Read the model definition and answer for the solid it produces. Units are mm, in the model's axes. Face numbers are marked on the shaded views. Coordinates: 2 decimals unless noted, no trailing zeros. Write each loop counter-clockwise with the first axis right and the second up, starting at its lowest first coordinate (ties: lowest second). Pieces come first, ordered by that corner, then holes. Notation, with made-up numbers: (0, 2) - (7, 2) arc R10 ccw to (7, 15) - close; hole circle Ø4 at (-37.5, 27). An arc over 180 degrees is marked (long way). Return JSON: item names as keys, results as strings.
```python
from build123d import *

# Parameters (mm, degrees)
SKETCH_1_R      = 5.5
EXTRUDE_1_DEPTH = 1.5
SKETCH_2_R      = 2.5
EXTRUDE_2_DEPTH = 2
SKETCH_3_R      = 10.188778254
EXTRUDE_3_DEPTH = 20
FILLET_2_R      = 2
FILLET_3_R      = 2
SCALE_1_SCALE   = 1.703703703


with BuildPart() as part:
    # 草图1 → 凸台-拉伸1 (new body)
    with BuildSketch(Plane(origin=(0, 0, 0), x_dir=(1, 0, 0), z_dir=(0, 1, 0))):
        with Locations(Location((0, 0, 0), (0, 0, 270))):
            Circle(SKETCH_1_R)
    extrude(amount=EXTRUDE_1_DEPTH)

    # 草图2 → 凸台-拉伸2 (add)
    with BuildSketch(Plane(origin=(0, 1.5, 0), x_dir=(1, 0, 0), z_dir=(0, 1, 0))):
        with Locations(Location((0, 0, 0), (0, 0, 270))):
            Circle(SKETCH_2_R)
    extrude(amount=EXTRUDE_2_DEPTH)

    # 草图3 → 凸台-拉伸3 (add)
    with BuildSketch(Plane(origin=(0, 3.5, 0), x_dir=(1, 0, 0), z_dir=(0, 1, 0))):
        with Locations(Location((0, 0, 0), (0, 0, 270))):
            Circle(SKETCH_3_R)
    extrude(amount=EXTRUDE_3_DEPTH)

    # 圆角2
    fillet_2_edges = [part.edges().sort_by_distance(p)[0] for p in [
        (0, 23.5, -10.188778254),
    ]]
    fillet(fillet_2_edges, radius=FILLET_2_R)

    # 圆角3
    fillet_3_edges = [part.edges().sort_by_distance(p)[0] for p in [
        (0, 3.5, -2.5),
        (0, 3.5, -10.188778254),
    ]]
    fillet(fillet_3_edges, radius=FILLET_3_R - 0.0001)  # a hair under: the kernel refuses the full size


with BuildPart() as part_1:
    # 缩放比例1: scaled about (0, 13.134921616, 0)
    add(part.part.scale(SCALE_1_SCALE).moved(Location((0, -9.243092979, 0))))


solid = part_1.part
```
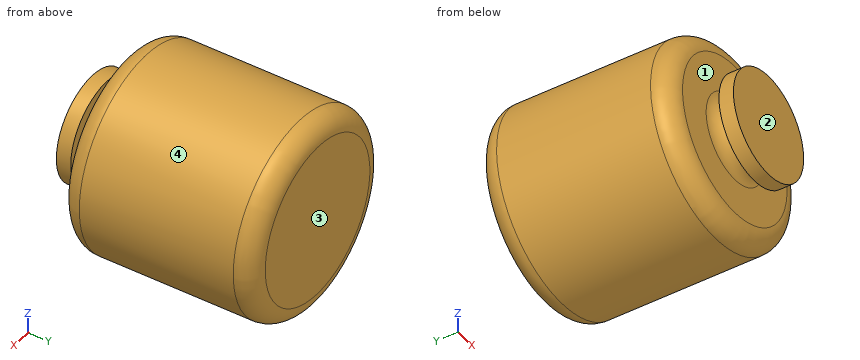
(1) A cutting plane is placed at D-D (y = -1). Determine the outline of the cut face in (x, z).
Answer:
{"outline": "circle Ø34.33 at (0, 0)"}
(2) A cutting plane is placed at C-C (y = 5). Determine the outline of the cut face in (x, z).
Answer:
{"outline": "circle Ø34.72 at (0, 0)"}
(3) Determine the mould class of the marked faces 1, 2, 3 and 4 for opening direction Y: +Y half, -Y half, draft (parallel to the pull), parting line (faces both ways), or undercut.
Answer:
{"face 1": "undercut", "face 2": "-Y half", "face 3": "+Y half", "face 4": "draft"}
(4) Straight lines are drawn through the part: line 1 (Y direction, x = 9, z = -0.5); line 2 (Y direction, x = 12.5, z = -1.5); line 3 (Y direction, x = 5, z = -3.5). For each, find the intervals that lie inside material, in ascending order. Write a range as from..to.
Answer:
{"line 1": "-9.24..-6.69, -3.28..30.79", "line 2": "-3.28..30.79", "line 3": "-9.24..-6.69, -3.66..30.79"}
(5) Flat-ended cylindrical pins translate along their axes: P1, Ø2, axis at y = 1, z = 10, coming from the +X side; P2, Ø8, axis at x = 10.5, y = 7, coming from the -Z side; P3, Ø1, axis at x = 3.5, y = 19.5, coming from the -Z side. Find the tip coordinate at first contact, or state that the pin passes through.
Answer:
{"P1": "x = 14.84", "P2": "z = -16.1", "P3": "z = -17.1"}
